The listing builds one solid part. Answer for the finished solid, in the listing's coordinates (mm). Coordinates: 2 decimals unless noted, no trailing zeros. Order: outer loops, then holes, each group sorted by start corner. A loop starts at its lowest first (then second) coordinate and runs counter-clockwise, first axis right, second up. Notation, with made-up numbers: (-17.5, 81) -> (1.5, 81) arc R10 ccw to (1.5, 99) -> close; hole circle Ø6 at (6, 79.25). An arc over 180 degrees is marked (long way). Return JSON: item names as keys, results as strings.
from build123d import *

# Parameters (mm, degrees)
SKETCH1_W           = 323.85
SKETCH1_H           = 203.2
BOSS_EXTRUDE1_DEPTH = 15.875
SKETCH2_W           = 292.1
SKETCH2_H           = 165.1
CUT_EXTRUDE1_DEPTH  = 2.54
SKETCH3_R           = 2.3749
CUT_EXTRUDE2_DEPTH  = 2.54


with BuildPart() as part:
    # Sketch1 → Boss-Extrude1 (new body)
    with BuildSketch(Plane.XY):
        Rectangle(SKETCH1_W, SKETCH1_H)
    extrude(amount=BOSS_EXTRUDE1_DEPTH)

    # Sketch2 → Cut-Extrude1 (cut)
    with BuildSketch(Plane.XY.offset(15.875)):
        Rectangle(SKETCH2_W, SKETCH2_H)
    extrude(amount=-CUT_EXTRUDE1_DEPTH, mode=Mode.SUBTRACT)

    # Sketch3 → Cut-Extrude2 (cut)
    with BuildSketch(Plane(origin=(0, 0, 0), x_dir=(-1, 0, 0), z_dir=(0, 0, -1))):
        with Locations((-37.5, 37.5)):
            Circle(SKETCH3_R)
        with Locations((37.5, 37.5)):
            Circle(SKETCH3_R)
        with Locations((37.5, -37.5)):
            Circle(SKETCH3_R)
        with Locations((-37.5, -37.5)):
            Circle(SKETCH3_R)
    extrude(amount=-CUT_EXTRUDE2_DEPTH, mode=Mode.SUBTRACT)


solid = part.part
1. The part is cut by section B-B on y = -20. Give the vertices of the cut face in (x, z) (3 decimals), and give its area (3 significant figures).
Answer block:
{"outline": "(-161.925, 0) -> (161.925, 0) -> (161.925, 15.875) -> (146.05, 15.875) -> (146.05, 13.335) -> (-146.05, 13.335) -> (-146.05, 15.875) -> (-161.925, 15.875) -> close", "area": "4,400 mm2"}
2. Each of these flat-tipped pins is pushed along its axis until it touches: pin 1 Ø5 at (x, y) = (37, 65) entering from +Z (3 decimals); pin 2 Ø2.5 at (x, y) = (-37.5, 36.5) entering from -Z. Where does it stop, or does it pass through?
Answer block:
{"pin 1": "stops at z = 13.335", "pin 2": "stops at z = 2.54"}
3. The part is cut by section A-A on x = -88.5. Give the vertices of the cut face in (y, z) (3 decimals).
Answer block:
{"outline": "(-101.6, 0) -> (101.6, 0) -> (101.6, 15.875) -> (82.55, 15.875) -> (82.55, 13.335) -> (-82.55, 13.335) -> (-82.55, 15.875) -> (-101.6, 15.875) -> close"}
4. Consider line 1 (Y direction, x = 37.5, z = 2); line 2 (Y direction, x = -24.5, z = 13.5); line 3 (X direction, y = 23, z = 14.75) (3 decimals). Determine where each line is inside the solid, lowest interval first. Write a range as from..to.
Answer block:
{"line 1": "y = -101.6..-39.87, -35.13..35.13, 39.87..101.6", "line 2": "y = -101.6..-82.55, 82.55..101.6", "line 3": "x = -161.925..-146.05, 146.05..161.925"}
5. Determine the mould class of faces 1 (the face through (-2, -101.6, 8)), 2 (the face through (-2, 1, 13.335)), 3 (the face through (-2, 1, 0)) for opening direction Y: pulls with the +Y half, pulls with the -Y half, needs draft (parallel to the pull), parting line crosses it, or undercut.
Answer block:
{"face 1": "pulls with the -Y half", "face 2": "undercut", "face 3": "needs draft"}
